```python
from build123d import *

# Parameters (mm, degrees)
BASE_FLANGE2_DEPTH         = 475
SKETCH13_R                 = 2.25
CUT_EXTRUDE4_DEPTH         = 619.939427235
SKETCH14_R                 = 11.5
SKETCH14_R_2               = 1.75
STEPPER_MOTOR_CUTOUT_DEPTH = 0.889
SKETCH15_R                 = 2.25
CUT_EXTRUDE6_DEPTH         = 0.889
SKETCH16_W                 = 46.8
SKETCH16_H                 = 27
CUT_EXTRUDE7_DEPTH         = 0.889
M4_CLEARANCE_HOLE1_D       = 4.5
EDGE_FLANGE1_DEPTH         = 50.8
EDGE_FLANGE1_BEND_DEPTH    = 366.29983991
EDGE_FLANGE1_BEND_2_DEPTH  = 50.8
BREAK_CORNER1_START        = 475.381
BREAK_CORNER1_DEPTH        = 0.889
CUT_EXTRUDE8_DEPTH         = 10
M4_CLEARANCE_HOLE2_D       = 4.5
M4_CLEARANCE_HOLE3_D       = 4.5


# Read off the part's stored shape, not the designer's step: Break-Corner1
# Sheet-metal steps are written as plain solids
with BuildPart() as part:
    # Sketch1 → Base-Flange2 (new body)
    with BuildSketch(Plane(origin=(0, 0, 0), x_dir=(1, 0, 0), z_dir=(0, 1, 0))):
        with BuildLine():
            Line((195.849919955, 63.5), (195.849919955, 12.7))
            ThreePointArc((195.849919955, 12.7), (192.130176076, 3.719743879), (183.149919955, 0))
            Line((183.149919955, 0), (-183.149919955, 0))
            ThreePointArc((-183.149919955, 0), (-192.130176076, 3.719743879), (-195.849919955, 12.7))
            Line((-195.849919955, 12.7), (-195.849919955, 63.5))
            Line((-195.849919955, 63.5), (-194.960919955, 63.5))
            Line((-194.960919955, 63.5), (-194.960919955, 12.7))
            ThreePointArc((-194.960919955, 12.7), (-191.501558148, 4.348361807), (-183.149919955, 0.889))
            Line((-183.149919955, 0.889), (183.149919955, 0.889))
            ThreePointArc((183.149919955, 0.889), (191.501558148, 4.348361807), (194.960919955, 12.7))
            Line((194.960919955, 12.7), (194.960919955, 63.5))
            Line((194.960919955, 63.5), (195.849919955, 63.5))
        make_face()
    extrude(amount=BASE_FLANGE2_DEPTH)

    # Sketch13 → Cut-Extrude4 (cut, through all)
    with BuildSketch(Plane(origin=(195.849919955, 0, 0), x_dir=(0, 0, -1), z_dir=(1, 0, 0))):
        with Locations((50.096107, 60)):
            Circle(SKETCH13_R)
        with Locations((50.096107, 316.132840032)):
            Circle(SKETCH13_R)
        with Locations((50.096107, 30)):
            Circle(SKETCH13_R)
    extrude(amount=-CUT_EXTRUDE4_DEPTH, mode=Mode.SUBTRACT)

    # Sketch14 → Stepper motor cutout (cut)
    with BuildSketch(Plane.XY):
        with Locations((50, 311.73292)):
            Circle(SKETCH14_R)
        with Locations((34.5, 296.23292)):
            Circle(SKETCH14_R_2)
        with Locations((65.5, 296.23292)):
            Circle(SKETCH14_R_2)
        with Locations((34.5, 327.23292)):
            Circle(SKETCH14_R_2)
        with Locations((65.5, 327.23292)):
            Circle(SKETCH14_R_2)
        with Locations((-50, 311.73292)):
            Circle(SKETCH14_R)
        with Locations((-65.5, 296.23292)):
            Circle(SKETCH14_R_2)
        with Locations((-34.5, 296.23292)):
            Circle(SKETCH14_R_2)
        with Locations((-65.5, 327.23292)):
            Circle(SKETCH14_R_2)
        with Locations((-34.5, 327.23292)):
            Circle(SKETCH14_R_2)
    extrude(amount=-STEPPER_MOTOR_CUTOUT_DEPTH, mode=Mode.SUBTRACT)

    # Sketch15 → Cut-Extrude6 (cut)
    with BuildSketch(Plane.XY):
        with Locations((-145.753812955, 316.132839976)):
            Circle(SKETCH15_R)
        with Locations((-118.946026845, 316.132839976)):
            Circle(SKETCH15_R)
        with Locations((118.946026845, 316.132839976)):
            Circle(SKETCH15_R)
        with Locations((145.753812955, 316.132839976)):
            Circle(SKETCH15_R)
        with Locations((145.753812955, 59.61392)):
            Circle(SKETCH15_R)
        with Locations((118.946026845, 59.61392)):
            Circle(SKETCH15_R)
        with Locations((-118.946026845, 59.61392)):
            Circle(SKETCH15_R)
        with Locations((-145.753812955, 59.61392)):
            Circle(SKETCH15_R)
    extrude(amount=-CUT_EXTRUDE6_DEPTH, mode=Mode.SUBTRACT)

    # Sketch16 → Cut-Extrude7 (cut)
    with BuildSketch(Plane.XY):
        with Locations((-73.4, 23.5)):
            Rectangle(SKETCH16_W, SKETCH16_H)
    extrude(amount=-CUT_EXTRUDE7_DEPTH, mode=Mode.SUBTRACT)

    # M4 Clearance Hole1 (through all)
    with Locations(Plane.XY):
        with Locations((-75, 181.73292), (-75, 171.73292)):
            Hole(M4_CLEARANCE_HOLE1_D / 2)

    # Edge-Flange1 section (across the edge) → Edge-Flange1 (add)
    with BuildSketch(Plane(origin=(-194.960919955, 475.381, -63.5), x_dir=(0, -1, 0), z_dir=(0, 0, 1))):
        with BuildLine():
            Line((-0.889, 0.381), (-0.889, 9.111))
            Line((-0.889, 9.111), (0, 9.111))
            Line((0, 9.111), (0, 0.381))
            ThreePointArc((0, 0.381), (0.111592316, 0.111592316), (0.381, 0))
            Line((0.381, 0), (0.381, -0.889))
            ThreePointArc((0.381, -0.889), (-0.517025612, -0.517025612), (-0.889, 0.381))
        make_face()
    extrude(amount=EDGE_FLANGE1_DEPTH)

    # Edge-Flange1 section 2 (across the edge) → Edge-Flange1 bend (add)
    with BuildSketch(Plane(origin=(-183.149919955, 475.381, -0.889), x_dir=(0, -1, 0), z_dir=(1, 0, 0))):
        with BuildLine():
            Line((-0.889, 0.381), (-0.889, 9.111))
            Line((-0.889, 9.111), (0, 9.111))
            Line((0, 9.111), (0, 0.381))
            ThreePointArc((0, 0.381), (0.111592316, 0.111592316), (0.381, 0))
            Line((0.381, 0), (0.381, -0.889))
            ThreePointArc((0.381, -0.889), (-0.517025612, -0.517025612), (-0.889, 0.381))
        make_face()
    extrude(amount=EDGE_FLANGE1_BEND_DEPTH)

    # Edge-Flange1 section 3 (across the edge) → Edge-Flange1 bend 2 (add)
    with BuildSketch(Plane(origin=(194.960919955, 475.381, -12.7), x_dir=(0, -1, 0), z_dir=(0, 0, -1))):
        with BuildLine():
            Line((-0.889, 0.381), (-0.889, 9.111))
            Line((-0.889, 9.111), (0, 9.111))
            Line((0, 9.111), (0, 0.381))
            ThreePointArc((0, 0.381), (0.111592316, 0.111592316), (0.381, 0))
            Line((0.381, 0), (0.381, -0.889))
            ThreePointArc((0.381, -0.889), (-0.517025612, -0.517025612), (-0.889, 0.381))
        make_face()
    extrude(amount=EDGE_FLANGE1_BEND_2_DEPTH)

    # Break-Corner1 outline → Break-Corner1 (cut)
    with BuildSketch(Plane(origin=(0, 0, 0), x_dir=(1, 0, 0), z_dir=(0, 1, 0)).offset(BREAK_CORNER1_START)):
        Polygon((183.149919955, 10), (178.149919955, 10), (183.149919955, 5), align=None)
        Polygon((-183.149919955, 5), (-178.149919955, 10), (-183.149919955, 10), align=None)
        Polygon((185.849919955, 63.5), (185.849919955, 58.5), (190.849919955, 63.5), align=None)
        Polygon((190.849919955, 12.7), (185.849919955, 17.7), (185.849919955, 12.7), align=None)
        Polygon((-185.849919955, 63.5), (-190.849919955, 63.5), (-185.849919955, 58.5), align=None)
        Polygon((-185.849919955, 12.7), (-185.849919955, 17.7), (-190.849919955, 12.7), align=None)
    extrude(amount=BREAK_CORNER1_DEPTH, mode=Mode.SUBTRACT)

    # Sketch29 → Cut-Extrude8 (cut)
    with BuildSketch(Plane.XY):
        with BuildLine():
            Line((55, 416.73292), (105, 416.73292))
            ThreePointArc((105, 416.73292), (110, 411.73292), (105, 406.73292))
            Line((105, 406.73292), (55, 406.73292))
            ThreePointArc((55, 406.73292), (50, 411.73292), (55, 416.73292))
        make_face()
    extrude(amount=-CUT_EXTRUDE8_DEPTH, mode=Mode.SUBTRACT)

    # M4 Clearance Hole2 (through all)
    with Locations(Plane(origin=(0, 0, -0.889), x_dir=(-1, 0, 0), z_dir=(0, 0, -1))):
        with Locations((-13.403893, 275), (13.403893, 275), (13.403893, 59.61392)):
            Hole(M4_CLEARANCE_HOLE2_D / 2)

    # M4 Clearance Hole3 (through all)
    with Locations(Plane(origin=(0, 0, -0.889), x_dir=(-1, 0, 0), z_dir=(0, 0, -1))):
        with Locations((-106.393607124, 300), (-87.343607124, 300)):
            Hole(M4_CLEARANCE_HOLE3_D / 2)


solid = part.part
```
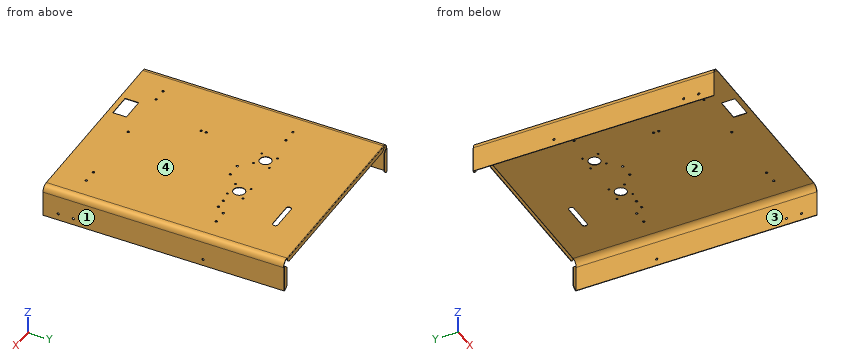
The model under review builds one solid part; all positions refer to its coordinate system, in mm. Face numbers are marked on the shaded views. Round coordinates to 2 decimals unless told otherwise and drop trailing zeros. Loops run counter-clockwise (first coordinate to the right, second up) from the corner with the lowest first, then second, coordinate; pieces in that order, holes last. Notation, with made-up numbers: (41, 16) -> (83, 16) arc R11 ccw to (83, 22) -> close; hole circle Ø6 at (-28.75, -2). An arc over 180 degrees is marked (long way). Answer as a JSON object with one key per item and string values. Group by question number.
1) Mouldability with a two-part tool opening along X and no side actions: class the marked faces 1, 2, 3 and 4 as released by +X, released by -X, zero draft, split by the parting line, or undercut.
2) We need section A-A on z = -27.5. Write out the cut boundary in (x, y).
3) We need section B-B on x = 168. Write out the cut boundary in (y, z), then the cut area to 3 significant figures.
4) For pin 1 Ø10 at (x, y) = (4.5, 57.5) entering from -Z; pin 2 Ø1.4 at (y, z) = (475.5, -3) entering from +X, all flat-tipped, find the tip position at first contact; note any pin that passes through.
5) We need section C-C on y = 229. Write out the cut boundary in (x, z), then the cut area to 3 significant figures.
6) For line 1 (X direction, y = 149, z = -29.5); line 2 (X direction, y = 386.5, z = -11); line 3 (Z direction, x = -51, y = 195), list the stretches that pass through material, from the lowest coordinate up. Write a range as [from, to].
Result set:
{
 "1": {"face 1": "released by +X", "face 2": "undercut", "face 3": "undercut", "face 4": "zero draft"},
 "2": {"outline": "(-195.85, 0) -> (-194.96, 0) -> (-194.96, 475) arc R0.38 cw to (-194.58, 475.38) -> (-185.85, 475.38) -> (-185.85, 476.27) -> (-194.58, 476.27) arc R1.27 ccw to (-195.85, 475) -> close; (185.85, 475.38) -> (194.58, 475.38) arc R0.38 cw to (194.96, 475) -> (194.96, 0) -> (195.85, 0) -> (195.85, 475) arc R1.27 ccw to (194.58, 476.27) -> (185.85, 476.27) -> close"},
 "3": {"outline": "(0, -0.89) -> (475, -0.89) arc R0.38 cw to (475.38, -1.27) -> (475.38, -10) -> (476.27, -10) -> (476.27, -1.27) arc R1.27 ccw to (475, 0) -> (0, 0) -> close", "area": "431 mm²"},
 "4": {"pin 1": "z = -0.89", "pin 2": "x = 191.89"},
 "5": {"outline": "(-195.85, -63.5) -> (-194.96, -63.5) -> (-194.96, -12.7) arc R11.81 cw to (-183.15, -0.89) -> (183.15, -0.89) arc R11.81 cw to (194.96, -12.7) -> (194.96, -63.5) -> (195.85, -63.5) -> (195.85, -12.7) arc R12.7 ccw to (183.15, 0) -> (-183.15, 0) arc R12.7 ccw to (-195.85, -12.7) -> close", "area": "450 mm²"},
 "6": {"line 1": "[-195.85, -194.96], [194.96, 195.85]", "line 2": "[-195.74, -194.84], [194.84, 195.74]", "line 3": "[-0.89, 0]"}
}
